Could you check a few things on this model? Use its own coordinates, in mm. A direction names the side the tool comes from. Give positions to 0.01 mm unless a question says otherwise; leave off trailing zeros. Order: outer loops, then holes, each group sorted by start corner. A loop starts at its lowest first (then second) coordinate and runs counter-clockwise, first axis right, second up.
(1) On a 3-axis mill with a long thin cutter (end or side, diameter ignored), from which of +Z, -Z, +X, -X, +Y, -Y can I reach the whole of each face in a straight line? I mean faces 1 (the flat face through (1, 9, -0.8)), 2 (the flat face through (1, 6.7, -4)), 3 (the flat face through (1, 11.7, -4)). Say none if no direction works.
(2) Imagine slicing it at A-A, the plane z = -1. Write out the boundary of the cut face in (x, y).
(3) If I drill on probe 1 along Z at (x, y) = (1.75, 8.25); probe 2 along Y at (x, z) = (1.4, -2.75); probe 3 along X at (y, z) = (4.5, -1), over which ranges is the centre line in solid material (lowest first)?
(4) Will these pins go through, and if not, where does the flat tip stop? pin 1 (1 mm diameter, centred on y = 0.5, z = -4, fed in from +X); pin 2 (0.9 mm diameter, centred on x = 0.5, y = -0.5, fed in from -Z); pin 3 (1 mm diameter, centred on x = 1.5, z = -3.5, fed in from -Y).
(5) Imagine slicing it at C-C, the plane x = 1. Write out the boundary of the cut face in (y, z), then the cut area to 3 significant figures.
(6) Imagine slicing it at B-B, the plane y = 9.25. Write out the boundary of the cut face in (x, z).
(7) Imagine slicing it at D-D, the plane y = 1.5. Write out the boundary of the cut face in (x, z), then the cut area to 3 significant figures.
from build123d import *

# Parameters (mm, degrees)
RESSALTO_EXTRUS_O1_DEPTH = 0.8
ESBO_O2_W                = 6.4
ESBO_O2_H                = 5
RESSALTO_EXTRUS_O2_DEPTH = 1.2


with BuildPart() as part:
    # Esboço1 → Ressalto-extrusão1 (new body)
    with BuildSketch(Plane(origin=(0, 0, 0), x_dir=(0, 0, -1), z_dir=(1, 0, 0))):
        Polygon((0, 0), (1.5, 0), (1.5, -0.8), (6.5, -0.8), (6.5, 0), (8, 0), (8, 12.5), (0, 12.5), align=None)
    extrude(amount=RESSALTO_EXTRUS_O1_DEPTH)

    # Esboço2 → Ressalto-extrusão2 (add)
    with BuildSketch(Plane(origin=(0.8, 0, 0), x_dir=(0, 0, -1), z_dir=(1, 0, 0))):
        with Locations((4, 9.2)):
            Rectangle(ESBO_O2_W, ESBO_O2_H)
    extrude(amount=RESSALTO_EXTRUS_O2_DEPTH)


solid = part.part
Answer block:
1. face 1: +Z, +X, +Y, -Y
1. face 2: +Z, -Z, +X, -Y
1. face 3: +Z, -Z, +X, +Y
2. outline: (0, 0) - (0.8, 0) - (0.8, 6.7) - (2, 6.7) - (2, 11.7) - (0.8, 11.7) - (0.8, 12.5) - (0, 12.5) - close
3. probe 1: z = -7.2 to -0.8
3. probe 2: y = 6.7 to 11.7
3. probe 3: x = 0 to 0.8
4. pin 1: stops at x = 0.8
4. pin 2: stops at z = -6.5
4. pin 3: stops at y = 6.7
5. outline: (6.7, -7.2) - (11.7, -7.2) - (11.7, -0.8) - (6.7, -0.8) - close
5. area: 32.0 mm2
6. outline: (0, -8) - (0.8, -8) - (0.8, -7.2) - (2, -7.2) - (2, -0.8) - (0.8, -0.8) - (0.8, 0) - (0, 0) - close
7. outline: (0, -8) - (0.8, -8) - (0.8, 0) - (0, 0) - close
7. area: 6.40 mm2
